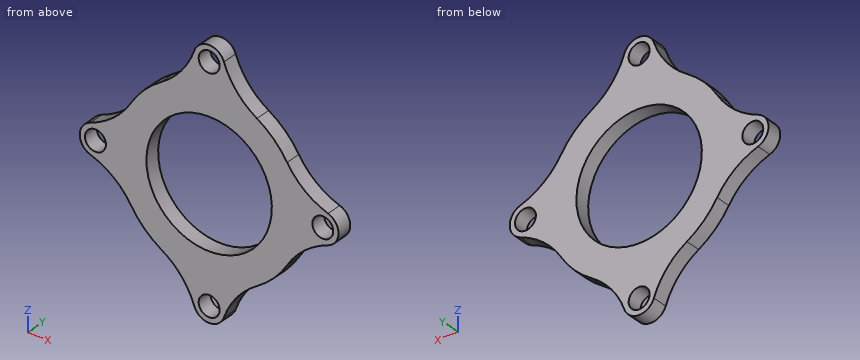
from build123d import *

# Parameters (mm, degrees)
SKETCH_1_R      = 12
SKETCH_1_R_2    = 2
EXTRUDE_1_DEPTH = 3


with BuildPart() as part:
    # ｽｹｯﾁ1 → ﾎﾞｽ - 押し出し1 (new body)
    with BuildSketch(Plane(origin=(0, 0, 0), x_dir=(1, 0, 0), z_dir=(0, 1, 0))):
        with BuildLine():
            ThreePointArc((-9.145896655, 14.919871795), (-12.374368671, 12.374368671), (-14.919871795, 9.145896655))
            ThreePointArc((-14.919871795, 9.145896655), (-18.286619233, 5.313420016), (-22.743055556, 2.830872774))
            ThreePointArc((-22.743055556, 2.830872774), (-24.75, 0), (-22.743055556, -2.830872774))
            ThreePointArc((-22.743055556, -2.830872774), (-18.286619233, -5.313420016), (-14.919871795, -9.145896655))
            ThreePointArc((-14.919871795, -9.145896655), (-12.374368671, -12.374368671), (-9.145896655, -14.919871795))
            ThreePointArc((-9.145896655, -14.919871795), (-5.313420016, -18.286619233), (-2.830872774, -22.743055556))
            ThreePointArc((-2.830872774, -22.743055556), (0, -24.75), (2.830872774, -22.743055556))
            ThreePointArc((2.830872774, -22.743055556), (5.313420016, -18.286619233), (9.145896655, -14.919871795))
            ThreePointArc((9.145896655, -14.919871795), (12.374368671, -12.374368671), (14.919871795, -9.145896655))
            ThreePointArc((14.919871795, -9.145896655), (18.286619233, -5.313420016), (22.743055556, -2.830872774))
            ThreePointArc((22.743055556, -2.830872774), (24.75, 0), (22.743055556, 2.830872774))
            ThreePointArc((22.743055556, 2.830872774), (18.286619233, 5.313420016), (14.919871795, 9.145896655))
            ThreePointArc((14.919871795, 9.145896655), (12.374368671, 12.374368671), (9.145896655, 14.919871795))
            ThreePointArc((9.145896655, 14.919871795), (5.313420016, 18.286619233), (2.830872774, 22.743055556))
            ThreePointArc((2.830872774, 22.743055556), (0, 24.75), (-2.830872774, 22.743055556))
            ThreePointArc((-2.830872774, 22.743055556), (-5.313420016, 18.286619233), (-9.145896655, 14.919871795))
        make_face()
        with Locations(Location((0, 0, 0), (0, 0, 270))):
            Circle(SKETCH_1_R, mode=Mode.SUBTRACT)
        with Locations(Location((0, 21.75, 0), (0, 0, 270))):
            Circle(SKETCH_1_R_2, mode=Mode.SUBTRACT)
        with Locations(Location((21.75, 0, 0), (0, 0, 270))):
            Circle(SKETCH_1_R_2, mode=Mode.SUBTRACT)
        with Locations(Location((0, -21.75, 0), (0, 0, 270))):
            Circle(SKETCH_1_R_2, mode=Mode.SUBTRACT)
        with Locations(Location((-21.75, 0, 0), (0, 0, 270))):
            Circle(SKETCH_1_R_2, mode=Mode.SUBTRACT)
    extrude(amount=EXTRUDE_1_DEPTH)


solid = part.part
Source: CAD feature listing. Evaluate the final solid. Frame: model axes, mm. Round coordinates to 2 decimals unless told otherwise and drop trailing zeros. Loops run counter-clockwise (first coordinate to the right, second up) from the corner with the lowest first, then second, coordinate; pieces in that order, holes last. Notation, with made-up numbers: (18.25, 27) - (54.25, 27) arc R12 cw to (54.25, 44) - close; hole circle Ø2 at (-19.5, -23.5). An arc over 180 degrees is marked (long way). Write item = value, one per line. Start each with the question number.
Item 1: Section query A-A on x = 21. Output: boundary loops of the cut face in (y, z).
Item 2: Section query B-B on y = 0.7. Output: boundary loops of the cut face in (x, z), plus the area to 3 significant figures.
Item 3: Section query D-D on x = 15.5. Output: boundary loops of the cut face in (y, z).
Item 4: Material intervals for line 1 (X direction, y = 1.4, z = 0); line 2 (Z direction, x = 5, y = 2.2); line 3 (Z direction, x = 20.5, y = 2.8), sorted ascending.
Item 5: Section query C-C on z = -5.5. Output: boundary loops of the cut face in (x, y).
Item 6: First-contact query: pin 1 Ø1.5 at (x, y) = (-17.5, 2) entering from +Z; pin 2 Ø1.5 at (x, y) = (2, 2) entering from +Z; pin 3 Ø1 at (x, y) = (-14, 2) entering from -Z. Flat tips, straight axial feed; report the tip coordinate or a pass-through.
Results list:
q1.outline = (0, -3.57) - (3, -3.57) - (3, -1.85) - (0, -1.85) - close; (0, 1.85) - (3, 1.85) - (3, 3.57) - (0, 3.57) - close
q2.outline = (-22.74, -2.83) arc R15 cw to (-14.92, -9.15) arc R17.5 ccw to (-9.15, -14.92) arc R15 cw to (-2.83, -22.74) arc R3 ccw to (2.83, -22.74) arc R15 cw to (9.15, -14.92) arc R17.5 ccw to (14.92, -9.15) arc R15 cw to (22.74, -2.83) arc R3 ccw to (22.74, 2.83) arc R15 cw to (14.92, 9.15) arc R17.5 ccw to (9.15, 14.92) arc R15 cw to (2.83, 22.74) arc R3 ccw to (-2.83, 22.74) arc R15 cw to (-9.15, 14.92) arc R17.5 ccw to (-14.92, 9.15) arc R15 cw to (-22.74, 2.83) arc R3 ccw to start; hole circle Ø4 at (-21.75, 0); hole circle Ø24 at (0, 0); hole circle Ø4 at (0, -21.75); hole circle Ø4 at (0, 21.75); hole circle Ø4 at (21.75, 0)
q2.area = 693 mm²
q3.outline = (0, -8.27) - (3, -8.27) - (3, 8.27) - (0, 8.27) - close
q4.line_1 = -24.75 to -23.75, -19.75 to -12, 12 to 19.75, 23.75 to 24.75
q4.line_2 = -18.69 to -10.91, 10.91 to 18.69
q4.line_3 = -3.83 to -1.56, 1.56 to 3.83
q5.outline = (-18.06, 0) - (-10.67, 0) - (-10.67, 3) - (-18.06, 3) - close; (10.67, 0) - (18.06, 0) - (18.06, 3) - (10.67, 3) - close
q6.pin_1 = 6.74
q6.pin_2 = 24.48
q6.pin_3 = -11.14
